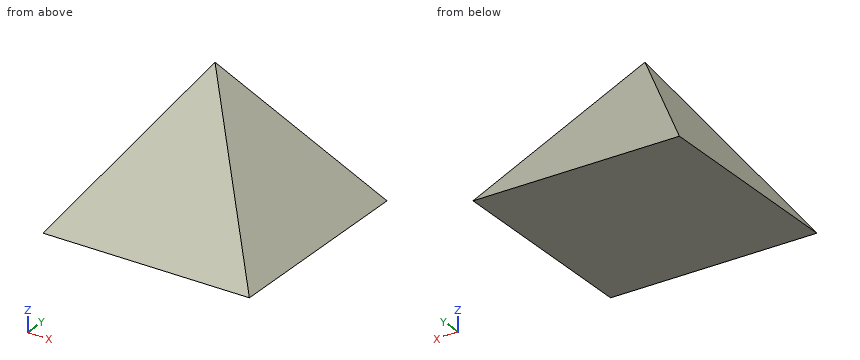
Solid Edge part; units mm, degrees
sketch "Sketch1" plane through (0, 0, 0) normal (0, -1, 0) x (1, 0, 0)
  arc A0 (-75, 0) -> (0, 75) centre (0, 0) cw
  line L0 (0, 0) -> (0, 75)
  line L1 (-75, 0) -> (0, 0)
revolve "RevolvedProtrusion1" add sketch "Sketch1" angle 360 about axis through (0, 0, 0) along (0, 0, 1)
sketch "Sketch2" plane through (0, 0, 0) normal (0, -1, 0) x (1, 0, 0)
  line L0 (0, 35.3553) -> (25, 0)
  line L1 (0, 35.3553) -> (-25, 0)
extrude "Cutout1" cut sketch "Sketch2" along normal through all and the other way through all material side at (12.5408, 0, 17.7065)
pattern_circular "Pattern1" count 4 over 360 about axis through (0, 0, 0) along (0, 0, 1) of "Cutout1"
The model under review builds one solid part; all positions refer to its coordinate system, in mm. Round coordinates to 2 decimals unless told otherwise and drop trailing zeros. Loops run counter-clockwise (first coordinate to the right, second up) from the corner with the lowest first, then second, coordinate; pieces in that order, holes last. Notation, with made-up numbers: (13.5, -36) -> (60.5, -36) arc R29 ccw to (60.5, -11) -> close; hole circle Ø6 at (4, 44.5). An arc over 180 degrees is marked (long way). Write item = value, one per line. Start each with the question number.
Item 1: To check wall thickness, follow L1, parallel to Z at x = -1, y = -5; L2, parallel to Y at x = -10, z = 2.5; L3, parallel to X at y = -13, z = 4.5. State the ranges of each line that lie inside material, in increasing order.
Item 2: Take a section at B-B on y = -18. Give the boundary of the cut face in (x, z).
Item 3: Take a section at A-A on z = 12.5. Give the boundary of the cut face in (x, y).
Item 4: Insertion check: pin 1 (6 mm diameter, centred on x = 8, z = 24, fed in from +Y); pin 2 (8 mm diameter, centred on y = -7.5, z = 28.5, fed in from +X); pin 3 (1 mm diameter, centred on y = 3, z = 28.5, fed in from -X); pin 4 (1 mm diameter, centred on x = -9.5, y = -17, fed in from -Z). Each pin has a flat end and moves straight along its axis. Give the tip position at first contact, or say it passes through.
Result:
q1.L1 = 0 to 28.28
q1.L2 = -23.23 to 23.23
q1.L3 = -21.82 to 21.82
q2.outline = (-25, 0) -> (25, 0) -> (18, 9.9) -> (-18, 9.9) -> close
q3.outline = (-16.16, -16.16) -> (16.16, -16.16) -> (16.16, 16.16) -> (-16.16, 16.16) -> close
q4.pin_1 = 10.15
q4.pin_2 = 7.68
q4.pin_3 = -5.2
q4.pin_4 = 0
